Input: part model. Units: mm. Frame: model coordinates. A direction names the side the tool comes from. Round coordinates to 2 decimals unless told otherwise and drop trailing zeros. Write each loop counter-clockwise with the first axis right and the second up, starting at its lowest first coordinate (ties: lowest second). Pieces come first, ordered by that corner, then holes. Notation, with made-up numbers: (35.25, 46) -> (73.25, 46) arc R29 ccw to (73.25, 76) -> close; hole circle Ø11 at (-20.75, 69). An arc over 180 degrees is marked (long way). Use CSV: the item, a comma, the result in double quotes.
Autodesk Fusion 360 part; units mm, degrees
sketch "Sketch1" plane through (0, 0, 0) normal (0, 0, 1) x (1, 0, 0)
  line L0 (-14, 0) -> (175, 0)
  line L1 (180, -12) -> (180, 0)
  line L2 (178, 175) -> (-17, 175)
  line L3 (-19, 0) -> (-19, -12)
  line L4 (-19, -12) -> (-14, -12)
  line L5 (-14, -12) -> (-14, 0)
  line L6 (180, -12) -> (175, -12)
  line L7 (175, -12) -> (175, 0)
  line L8 (180, 0) -> (178, 0)
  line L9 (178, 0) -> (178, 175)
  line L10 (-17, 0) -> (-17, 175)
  line L11 (-17, 0) -> (-19, 0)
  dimension "d1" = 189
  dimension "d13" = 12
  dimension "d14" = 12
  dimension "d16" = 5
  dimension "d24" = 175
  dimension "d31" = 2
  dimension "d32" = 5
  dimension "d33" = 2
extrude "Extrude1" add sketch "Sketch1" along normal blind 10
sketch "Sketch2" plane through (-14, 0, 0) normal (1, 0, 0) x (0, 0, -1)
  line L0 (0, -12) -> (0, 0)
  line L1 (0, 0) -> (-10, 0)
  line L2 (-10, 0) -> (-10, -12)
  line L3 (-10, -12) -> (0, -12)
  circle A0 centre (-5, -5.6) radius 2.9
  dimension "d5" = 5.8
  dimension "d6" = 5.6
extrude "Extrude2" add sketch "Sketch2" along normal blind 10 contours A0
sketch "Sketch3" plane through (175, 0, 0) normal (-1, 0, 0) x (0, 0, 1)
  line L0 (0, 0) -> (0, -12)
  line L1 (0, -12) -> (10, -12)
  line L2 (10, -12) -> (10, 0)
  line L3 (10, 0) -> (0, 0)
  circle A0 centre (5, -5.6) radius 2.9
  dimension "d9" = 5.8
  dimension "d10" = 5.6
extrude "Extrude3" add sketch "Sketch3" along normal blind 10 contours A0
sketch "Sketch4" plane through (0, 0, 0) normal (0, 0, -1) x (-1, 0, 0)
  line L0 (19, -12) -> (19, 0)
  line L1 (17, 0) -> (17, 175)
  line L2 (17, 175) -> (-178, 175)
  line L3 (-178, 175) -> (-178, 0)
  line L4 (-178, 0) -> (-180, 0)
  line L5 (-180, 0) -> (-180, -12)
  line L6 (-180, -12) -> (-175, -12)
  line L7 (-175, -12) -> (-175, 0)
  line L8 (-175, 0) -> (14, 0)
  line L9 (14, 0) -> (14, -12)
  line L10 (14, -12) -> (19, -12)
  line L11 (-178, 0) -> (-180, 0)
  line L12 (-180, 0) -> (-180, -12)
  line L13 (-180, -12) -> (-175, -12)
  line L14 (-175, -12) -> (-175, 172)
  line L15 (-175, 172) -> (14, 172)
  line L16 (14, 172) -> (14, -12)
  line L17 (14, -12) -> (19, -12)
  line L18 (19, -12) -> (19, 0)
  line L19 (19, 0) -> (17, 0)
  line L20 (17, 0) -> (17, 175)
  line L21 (17, 175) -> (-178, 175)
  line L22 (-178, 175) -> (-178, 0)
  line L23 (19, 0) -> (17, 0)
  dimension "d19" = 3
  dimension "d20" = 3
  dimension "d21" = 3
extrude "Extrude4" add sketch "Sketch4" along normal blind 8 contours L0 L1 L2 L3 L4 L5 L6 L7 L9 L10 L11 L12 L13 L14 L15 L16 L17 L18 L19 L20 L21 L22 L23
fillet "Fillet1" radius 5 1 edges at (-16.5, -12, 10)
fillet "Fillet2" radius 5 1 edges at (177.5, -12, 10)
extrude "Extrude5" cut 1 faces at (112, 114.6667, 0) along direction (0, 0, 1) blind 2
Item 1: First-contact query: pin 1 Ø10 at (y, z) = (149, 3.5) entering from -X; pin 2 Ø3 at (x, y) = (136, 68) entering from -Z; pin 3 Ø1.6 at (x, z) = (-18, 5.5) entering from +Y. Flat tips, straight axial feed; report the tip coordinate or a pass-through.
Worked answers:
pin 1,"stops at x = -17"
pin 2,"stops at z = 2"
pin 3,"stops at y = 0"
Item 2: Pull-direction query (Y, two-part tool) for faces 1 (the face through (79, 175, 1)), 2 (the face through (170.07, -2.77, 4.37)), 3 (the face through (178, 89, 1)), 4 (the face through (-9.07, -2.77, 5.63)); classes: +Y half, -Y half, draft (parallel to the pull), parting line (faces both ways), or undercut.
Worked answers:
face 1,"+Y half"
face 2,"undercut"
face 3,"draft"
face 4,"undercut"
Item 3: Section query A-A on x = 89. Return the cut outline in (y, z), plus the area to 3 significant figures.
Worked answers:
outline,"(0, 2) -> (172, 2) -> (172, -8) -> (175, -8) -> (175, 10) -> (0, 10) -> close"
area,"1,430 mm²"
Item 4: Line query: line 1 (X direction, y = 164.5, z = -1.5); line 2 (X direction, y = -2, z = 5.25); line 3 (Z direction, x = 92, y = 63). Output: solid intervals per line, ascending.
Worked answers:
line 1,"x = -17 to -14, 175 to 178"
line 2,"x = -19 to -14, 175 to 180"
line 3,"z = 2 to 10"
Item 5: Section query B-B on y = 37.5. Return the cut outline in (x, z).
Worked answers:
outline,"(-17, -8) -> (-14, -8) -> (-14, 2) -> (175, 2) -> (175, -8) -> (178, -8) -> (178, 10) -> (-17, 10) -> close"
Item 6: Set-up query: faces 5 (the face through (-17, 86, 1)), 6 (the face through (82, 172, -3)), 7 (the face through (165, -6, 5)). Return all of +Z, -Z, +X, -X, +Y, -Y with unobstructed straight access to the full face (end or side cutting, diameter ignored); none if empty.
Worked answers:
face 5,"+Z, -Z, -X, +Y"
face 6,"-Z, -Y"
face 7,"+Z, -Z, -Y"
